from build123d import *

# Parameters (mm, degrees)
SKETCH1_W                  = 206
SKETCH1_H                  = 206
MAINBOSS_DEPTH             = 7
MAINBOSS_DRAFT             = -1
SKETCH4_R                  = 70
TRAYCUT_DEPTH              = 5
TRAYCUT_DRAFT              = -1
SKETCH5_R                  = 3
TRAYHOLE_DEPTH             = 7
TRAYHOLE_DRAFT             = -1
MAINFILLET_R               = 2
SKETCH6_R                  = 3
SHAFTHOLES_DEPTH           = 7
SHAFTHOLES_DRAFT           = -1
SKETCH6_R_2                = 5.5
SHAFTHOLES_PROFILE_2_DEPTH = 7
SHAFTHOLES_PROFILE_2_DRAFT = -1
SHAFTHOLES_PROFILE_3_DEPTH = 7
SHAFTHOLES_PROFILE_3_DRAFT = -1
SKETCH7_R                  = 1.5
BACKLEFTHOLDER_DEPTH       = 7
SKETCH8_R                  = 1.5
BACKRIGHTHOLDER_DEPTH      = 7
SKETCH9_R                  = 1.5
FRONTRIGHTHOLDER_DEPTH     = 7
SKETCH10_R                 = 1.5
FRONTLEFTHOLDER_DEPTH      = 7


with BuildPart() as part:
    # Sketch1 → MainBoss (with draft: the straight prism first)
    with BuildSketch(Plane(origin=(0, 0, 0), x_dir=(1, 0, 0), z_dir=(0, 1, 0))):
        Rectangle(SKETCH1_W, SKETCH1_H)
    extrude(amount=MAINBOSS_DEPTH)
    # MainBoss: the draft: its side faces are tilted about the plane it starts from
    mainboss_sides = [part.faces().sort_by_distance(p)[0] for p in [
        (-103, 3.5, 0),
        (0, 3.5, 103),
        (103, 3.5, 0),
        (0, 3.5, -103),
    ]]
    draft(mainboss_sides, Plane(origin=(0, 0, 0), x_dir=(1, 0, 0), z_dir=(0, 1, 0)), MAINBOSS_DRAFT)


with BuildPart() as traycut_tool:
    # Sketch4 → TrayCut (with draft: the straight prism first)
    with BuildSketch(Plane(origin=(0, 0, 0), x_dir=(-1, 0, 0), z_dir=(0, -1, 0))):
        with Locations((2, 27)):
            Circle(SKETCH4_R)
    extrude(amount=-TRAYCUT_DEPTH)
    # TrayCut: the draft: its side faces are tilted about the plane it starts from
    traycut_sides = [traycut_tool.faces().sort_by_distance(p)[0] for p in [
        (68, 2.5, -27),
    ]]
    draft(traycut_sides, Plane(origin=(0, 0, 0), x_dir=(-1, 0, 0), z_dir=(0, -1, 0)), TRAYCUT_DRAFT)


with BuildPart() as part_1:
    add(part.part)

    # TrayCut: cut by traycut_tool
    add(traycut_tool.part, mode=Mode.SUBTRACT)


with BuildPart() as trayhole_tool:
    # Sketch5 → TrayHole (with draft: the straight prism first)
    with BuildSketch(Plane.XZ.offset(-5)):
        with Locations((-2, -27)):
            Circle(SKETCH5_R)
    extrude(amount=-TRAYHOLE_DEPTH)
    # TrayHole: the draft: its side faces are tilted about the plane it starts from
    trayhole_sides = [trayhole_tool.faces().sort_by_distance(p)[0] for p in [
        (-5, 8.5, -27),
    ]]
    draft(trayhole_sides, Plane.XZ.offset(-5), TRAYHOLE_DRAFT)


with BuildPart() as part_2:
    add(part_1.part)

    # TrayHole: cut by trayhole_tool
    add(trayhole_tool.part, mode=Mode.SUBTRACT)

    # MainFillet
    mainfillet_edges = [part_2.edges().sort_by_distance(p)[0] for p in [
        (68, 0, -27),
        (-103, 0, 0),
        (0, 0, 103),
        (103, 0, 0),
        (0, 0, -103),
    ]]
    fillet(mainfillet_edges, radius=MAINFILLET_R)


with BuildPart() as shaftholes_tool:
    # Sketch6 → ShaftHoles (with draft: the straight prism first)
    with BuildSketch(Plane.XZ):
        with Locations((0.965394526, 76.05325216)):
            Circle(SKETCH6_R)
    extrude(amount=-SHAFTHOLES_DEPTH)
    # ShaftHoles: the draft: its side faces are tilted about the plane it starts from
    shaftholes_sides = [shaftholes_tool.faces().sort_by_distance(p)[0] for p in [
        (-2.034605474, 3.5, 76.05325216),
    ]]
    draft(shaftholes_sides, Plane.XZ, SHAFTHOLES_DRAFT)


with BuildPart() as part_3:
    add(part_2.part)

    # ShaftHoles: cut by shaftholes_tool
    add(shaftholes_tool.part, mode=Mode.SUBTRACT)


with BuildPart() as shaftholes_profile_2_tool:
    # Sketch6 → ShaftHoles profile 2 (with draft: the straight prism first)
    with BuildSketch(Plane.XZ):
        with Locations((-39.034601128, 76.034605474)):
            Circle(SKETCH6_R_2)
    extrude(amount=-SHAFTHOLES_PROFILE_2_DEPTH)
    # ShaftHoles profile 2: the draft: its side faces are tilted about the plane it starts from
    shaftholes_profile_2_sides = [shaftholes_profile_2_tool.faces().sort_by_distance(p)[0] for p in [
        (-44.534601128, 3.5, 76.034605474),
    ]]
    draft(shaftholes_profile_2_sides, Plane.XZ, SHAFTHOLES_PROFILE_2_DRAFT)


with BuildPart() as part_4:
    add(part_3.part)

    # ShaftHoles profile 2: cut by shaftholes_profile_2_tool
    add(shaftholes_profile_2_tool.part, mode=Mode.SUBTRACT)


with BuildPart() as shaftholes_profile_3_tool:
    # Sketch6 → ShaftHoles profile 3 (with draft: the straight prism first)
    with BuildSketch(Plane.XZ):
        with Locations((40.965394526, 76.05325216)):
            Circle(SKETCH6_R_2)
    extrude(amount=-SHAFTHOLES_PROFILE_3_DEPTH)
    # ShaftHoles profile 3: the draft: its side faces are tilted about the plane it starts from
    shaftholes_profile_3_sides = [shaftholes_profile_3_tool.faces().sort_by_distance(p)[0] for p in [
        (35.465394526, 3.5, 76.05325216),
    ]]
    draft(shaftholes_profile_3_sides, Plane.XZ, SHAFTHOLES_PROFILE_3_DRAFT)


with BuildPart() as part_5:
    add(part_4.part)

    # ShaftHoles profile 3: cut by shaftholes_profile_3_tool
    add(shaftholes_profile_3_tool.part, mode=Mode.SUBTRACT)

    # Sketch7 → BackLeftHolder (cut)
    with BuildSketch(Plane(origin=(0, 0, 0), x_dir=(-1, 0, 0), z_dir=(0, -1, 0))):
        with Locations(Location((98.034605474, -98.034605474, 0), (0, 0, 90))):
            Circle(SKETCH7_R)
    extrude(amount=-BACKLEFTHOLDER_DEPTH, mode=Mode.SUBTRACT)

    # Sketch8 → BackRightHolder (cut)
    with BuildSketch(Plane(origin=(0, 0, 0), x_dir=(-1, 0, 0), z_dir=(0, -1, 0))):
        with Locations(Location((-98.034605474, -98.034605474, 0), (0, 0, 90))):
            Circle(SKETCH8_R)
    extrude(amount=-BACKRIGHTHOLDER_DEPTH, mode=Mode.SUBTRACT)

    # Sketch9 → FrontRightHolder (cut)
    with BuildSketch(Plane(origin=(0, 0, 0), x_dir=(-1, 0, 0), z_dir=(0, -1, 0))):
        with Locations(Location((-98.034605474, 98.034605474, 0), (0, 0, 90))):
            Circle(SKETCH9_R)
    extrude(amount=-FRONTRIGHTHOLDER_DEPTH, mode=Mode.SUBTRACT)

    # Sketch10 → FrontLeftHolder (cut)
    with BuildSketch(Plane(origin=(0, 0, 0), x_dir=(-1, 0, 0), z_dir=(0, -1, 0))):
        with Locations(Location((98.034605474, 98.034605474, 0), (0, 0, 90))):
            Circle(SKETCH10_R)
    extrude(amount=-FRONTLEFTHOLDER_DEPTH, mode=Mode.SUBTRACT)


solid = part_5.part
The listing builds one solid part. Answer for the finished solid, in the listing's coordinates (mm). A direction names the side the tool comes from. Coordinates: 2 decimals unless noted, no trailing zeros. Write item = value, one per line. Start each with the question number.
1) A tool of negligible diameter and unlimited length cuts with its end or side. For faces 3 (the face through (-1, 5, -12)), 4 (the face through (21, 0, 43)), from which of +Z, -Z, +X, -X, +Y, -Y can it reach the whole face along a straight path? Write none if from no direction.
2) Straight lines are drawn through the part: line 1 (Z direction, x = -1, y = 3.75); line 2 (X direction, y = 6, z = 84); line 3 (Z direction, x = 81, y = 6.5). For each, find the intervals that lie inside material, in ascending order. Write a range as from..to.
3) The mould has two halves that part along Z. Classify faces 1 (the face through (40.257, 3.451, 81.447)), 2 (the face through (-1, 7, -1)): released by +Z, released by -Z, zero draft, split by the parting line, or undercut.
4) A cutting plane is placed at A-A (y = 3.5). Count the separate pieces of the cut face and the enclosed holes in it, then the cut area to 3 significant figures.
5) Given pin 1 Ø3 at (x, y) = (-13, 3.5) entering from -Z; pin 2 Ø1 at (y, z) = (5, 70.5) entering from +X; pin 3 Ø1 at (x, y) = (41, 5) entering from +Z; pin 4 Ø2.5 at (x, z) = (98.03, -98.03) entering from +Y, each flat-ended and moving along its own axis, determine where each tip first touches the part or whether it passes through.
Responses:
q1.face_3 = -Y
q1.face_4 = +Z, -Z, +X, -X, -Y
q2.line_1 = -103.07..-96.93, 42.93..73.87, 78.23..103.07
q2.line_2 = -103.1..103.1
q2.line_3 = -103.11..103.11
q3.face_1 = undercut
q3.face_2 = zero draft
q4.separate_pieces = 1
q4.enclosed_holes = 8
q4.area = 26,900 mm²
q5.pin_1 = -103.09
q5.pin_2 = 103.1
q5.pin_3 = 103.1
q5.pin_4 = through
